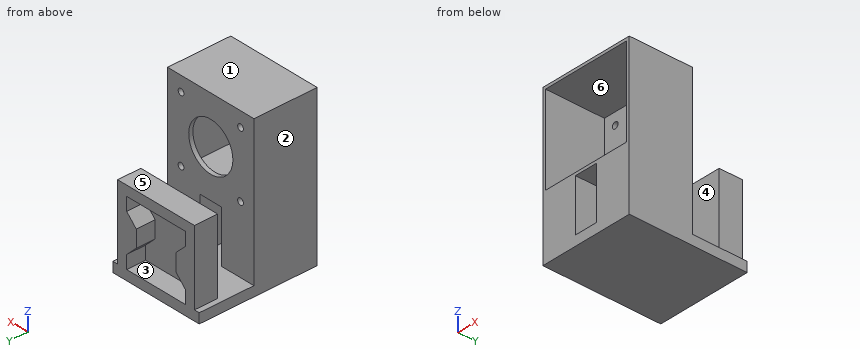
Solid Edge part; units mm, degrees
sketch "Sketch1" plane through (0, 0, 0) normal (0, -1, 0) x (1, 0, 0)
  line L0 (-20, -20) -> (20, -20)
  line L1 (20, -20) -> (20, 20)
  line L2 (20, 20) -> (-20, 20)
  line L3 (-20, 20) -> (-20, -20)
extrude "Protrusion1" add sketch "Sketch1" along normal mid plane 9
sketch "Sketch2" plane through (0, -4.5, 0) normal (0, -1, 0) x (1, 0, 0)
  line L0 (-15.3, -15.3) -> (15.3, -15.3)
  line L1 (15.3, -15.3) -> (15.3, -9)
  line L2 (10.3, -4) -> (15.3, -9)
  line L3 (10.3, 4) -> (10.3, -4)
  line L4 (10.3, 4) -> (15.3, 9)
  line L5 (15.3, 9) -> (15.3, 15.3)
  line L6 (15.3, 15.3) -> (-15.3, 15.3)
  line L7 (-15.3, 15.3) -> (-15.3, 9)
  line L8 (-10.3, 4) -> (-15.3, 9)
  line L9 (-10.3, 4) -> (-10.3, -4)
  line L10 (-10.3, -4) -> (-15.3, -9)
  line L11 (-15.3, -9) -> (-15.3, -15.3)
extrude "ExtrudedCutout_1" cut sketch "Sketch2" against normal blind 161.5
sketch "Sketch3" plane through (0, -21.5, 0) normal (0, -1, 0) x (0, 0, 1)
  line L0 (54.5, -22.5) -> (54.5, 22.5)
  line L1 (54.5, 22.5) -> (9.5, 22.5)
  line L2 (9.5, 22.5) -> (9.5, -22.5)
  line L3 (9.5, -22.5) -> (54.5, -22.5)
extrude "ExtrudedProtrusion_8" add sketch "Sketch3" along normal blind 30
sketch "Sketch4" plane through (0, -36.5, 32) normal (0, -1, 0) x (1, 0, 0)
  line L0 (-21.15, -21.15) -> (21.15, -21.15)
  line L1 (21.15, -21.15) -> (21.15, 21.15)
  line L2 (21.15, 21.15) -> (-21.15, 21.15)
  line L3 (-21.15, 21.15) -> (-21.15, -21.15)
extrude "ExtrudedCutout_4" cut sketch "Sketch4" against normal blind 13 and the other way blind 20
sketch "Sketch5" plane through (0, -23.5, 32) normal (0, -1, 0) x (0, 0, 1)
  circle A0 centre (0, 0) radius 11.5
  circle A1 centre (-15.5, 15.5) radius 1.5
  circle A2 centre (-15.5, -15.5) radius 1.5
  circle A3 centre (15.5, 15.5) radius 1.5
  circle A4 centre (15.5, -15.5) radius 1.5
extrude "Cutout1" cut sketch "Sketch5" against normal up to next
sketch "Sketch6" plane through (0, -4.5, 0) normal (0, -1, 0) x (1, 0, 0)
  line L0 (-20, 20) -> (20, 20)
  line L1 (20, 20) -> (20, -20)
  line L2 (20, -20) -> (-20, -20)
  line L3 (-20, -20) -> (-20, 20)
extrude "ExtrudedProtrusion_9" add sketch "Sketch6" along normal blind 2
sketch "Sketch7" plane through (0, -36.5, 9.5) normal (0, 0, -1) x (1, 0, 0)
  line L0 (-22.5, 15) -> (-22.5, -15)
  line L1 (-22.5, -15) -> (-5.5, -15)
  line L2 (-5.5, -15) -> (-5.5, 15)
  line L3 (-5.5, 15) -> (-22.5, 15)
  line L4 (22.5, 15) -> (22.5, -15)
  line L5 (22.5, -15) -> (5.5, -15)
  line L6 (5.5, -15) -> (5.5, 15)
  line L7 (5.5, 15) -> (22.5, 15)
extrude "ExtrudedProtrusion_13" add sketch "Sketch7" along normal blind 29
sketch "Sketch8" plane through (0, -1, -20) normal (0, 0, -1) x (0, -1, 0)
  line L0 (50.5, 22.5) -> (-5.5, 22.5)
  line L1 (-5.5, 22.5) -> (-5.5, -22.5)
  line L2 (-5.5, -22.5) -> (50.5, -22.5)
  line L3 (50.5, -22.5) -> (50.5, 22.5)
extrude "ExtrudedProtrusion_14" add sketch "Sketch8" against normal blind 4.7
For this review, take the finished solid that the model builds, in its own axes (mm). Face numbers are marked on the shaded views. A direction names the side the tool comes from. Give positions to 0.01 mm unless a question says otherwise; leave off trailing zeros. Order: outer loops, then holes, each group sorted by start corner. A loop starts at its lowest first (then second) coordinate and runs counter-clockwise, first axis right, second up.
1) Take a section at C-C (y = -42). Give the boundary of the cut face in (x, z), then the cut area to 3 significant figures.
2) Wall thickness on line 1 (Z direction, x = -15.5, y = -22.2); line 2 (Z direction, x = -2, y = -34); line 3 (X direction, y = -22.55, z = 47.5): over which ranges is each line inside the solid? List them lowest first.
3) Take a section at A-A (z = 47.5). Give the boundary of the cut face in (x, y).
4) Take a section at D-D (z = 32). Give the boundary of the cut face in (x, y), then the cut area to 3 significant figures.
5) The part is to be moulded in two halves that separate along X. For the marked faces 1, 2 and 3, say which applies: released by +X, released by -X, zero draft, split by the parting line, or undercut.
6) Insertion check: pin 1 (1.9 mm diameter, centred on y = -2, z = 13.5, fed in from +X); pin 2 (20.5 mm diameter, centred on x = 0, z = 32, fed in from -Y); pin 3 (9 mm diameter, centred on x = -5, z = 0.5, fed in from +Y); pin 4 (5 mm diameter, centred on y = -5.5, z = -6, fed in from -X). Each pin has a flat end and moves straight along its axis. Give the tip position at first contact, or say it passes through.
7) Take a section at B-B (x = 0). Give the boundary of the cut face in (y, z).
8) For the marked faces 4, 5 and 6, list the 3-axis set-ups (+Z, -Z, +X, -X, +Y, -Y) from which the entire face can be reached by the end or side of a thin tool; tool diameter is ignored.
Derived:
1. outline: (-22.5, -20) - (22.5, -20) - (22.5, 54.5) - (-22.5, 54.5) - close; hole (-21.15, 10.85) - (21.15, 10.85) - (21.15, 53.15) - (-21.15, 53.15) - close; hole (-5.5, -15.3) - (5.5, -15.3) - (5.5, 9.5) - (-5.5, 9.5) - close
1. area: 1,290 mm2
2. line 1: z = -20 to 15, 18 to 46, 49 to 54.5
2. line 2: z = -20 to -15.3, 9.5 to 10.85, 53.15 to 54.5
2. line 3: x = -22.5 to -17, -14 to 14, 17 to 22.5
3. outline: (-22.5, -51.5) - (-21.15, -51.5) - (-21.15, -23.5) - (-17, -23.5) - (-17, -21.5) - (-22.5, -21.5) - close; (-14, -23.5) - (14, -23.5) - (14, -21.5) - (-14, -21.5) - close; (17, -23.5) - (21.15, -23.5) - (21.15, -51.5) - (22.5, -51.5) - (22.5, -21.5) - (17, -21.5) - close
4. outline: (-22.5, -51.5) - (-21.15, -51.5) - (-21.15, -23.5) - (-11.5, -23.5) - (-11.5, -21.5) - (-22.5, -21.5) - close; (11.5, -23.5) - (21.15, -23.5) - (21.15, -51.5) - (22.5, -51.5) - (22.5, -21.5) - (11.5, -21.5) - close
4. area: 120 mm2
5. face 1: zero draft
5. face 2: released by -X
5. face 3: undercut
6. pin 1: stops at x = 20
6. pin 2: passes through
6. pin 3: stops at y = -4.5
6. pin 4: stops at x = -20
7. outline: (-51.5, -20) - (4.5, -20) - (4.5, -15.3) - (-4.5, -15.3) - (-4.5, 15.3) - (4.5, 15.3) - (4.5, 20) - (-6.5, 20) - (-6.5, -15.3) - (-51.5, -15.3) - close; (-51.5, 9.5) - (-21.5, 9.5) - (-21.5, 20.5) - (-23.5, 20.5) - (-23.5, 10.85) - (-51.5, 10.85) - close; (-51.5, 53.15) - (-23.5, 53.15) - (-23.5, 43.5) - (-21.5, 43.5) - (-21.5, 54.5) - (-51.5, 54.5) - close
8. face 4: +Z, +X, -X
8. face 5: +Z, +X, -X, +Y
8. face 6: -Y
